```python
from build123d import *

# Parameters (mm, degrees)
CROQUIS1_R     = 11
CROQUIS1_R_2   = 4
EXTRUIR1_DEPTH = 0.7
CROQUIS2_R     = 11
CROQUIS2_R_2   = 10.3
CROQUIS2_R_3   = 8.9
CROQUIS2_R_4   = 8.2
CROQUIS2_R_5   = 6.8
CROQUIS2_R_6   = 6.1
CROQUIS2_R_7   = 4.7
CROQUIS2_R_8   = 4
EXTRUIR2_DEPTH = 1.6
CROQUIS3_R     = 4.7
CROQUIS3_R_2   = 4
EXTRUIR3_DEPTH = 0.7


with BuildPart() as part:
    # Croquis1 → Extruir1 (new body)
    with BuildSketch(Plane(origin=(0, 0, 0), x_dir=(1, 0, 0), z_dir=(0, 1, 0))):
        with Locations(Location((0, 0, 0), (0, 0, 270))):
            Circle(CROQUIS1_R)
        with Locations(Location((0, 0, 0), (0, 0, 270))):
            Circle(CROQUIS1_R_2, mode=Mode.SUBTRACT)
    extrude(amount=EXTRUIR1_DEPTH)

    # Croquis2 → Extruir2 (add)
    # profile 1 of 4: a face of its own
    with BuildSketch(Plane(origin=(0, 0.7, 0), x_dir=(1, 0, 0), z_dir=(0, 1, 0))):
        with Locations(Location((0, 0, 0), (0, 0, 270))):
            Circle(CROQUIS2_R)
        with Locations(Location((0, 0, 0), (0, 0, 270))):
            Circle(CROQUIS2_R_2, mode=Mode.SUBTRACT)
    # profile 2 of 4: a face of its own
    with BuildSketch(Plane(origin=(0, 0.7, 0), x_dir=(1, 0, 0), z_dir=(0, 1, 0))):
        with Locations(Location((0, 0, 0), (0, 0, 270))):
            Circle(CROQUIS2_R_3)
        with Locations(Location((0, 0, 0), (0, 0, 270))):
            Circle(CROQUIS2_R_4, mode=Mode.SUBTRACT)
    # profile 3 of 4: a face of its own
    with BuildSketch(Plane(origin=(0, 0.7, 0), x_dir=(1, 0, 0), z_dir=(0, 1, 0))):
        with Locations(Location((0, 0, 0), (0, 0, 270))):
            Circle(CROQUIS2_R_5)
        with Locations(Location((0, 0, 0), (0, 0, 270))):
            Circle(CROQUIS2_R_6, mode=Mode.SUBTRACT)
    # profile 4 of 4: a face of its own
    with BuildSketch(Plane(origin=(0, 0.7, 0), x_dir=(1, 0, 0), z_dir=(0, 1, 0))):
        with Locations(Location((0, 0, 0), (0, 0, 270))):
            Circle(CROQUIS2_R_7)
        with Locations(Location((0, 0, 0), (0, 0, 270))):
            Circle(CROQUIS2_R_8, mode=Mode.SUBTRACT)
    extrude(amount=EXTRUIR2_DEPTH)

    # Croquis3 → Extruir3 (add)
    with BuildSketch(Plane(origin=(0, 2.3, 0), x_dir=(1, 0, 0), z_dir=(0, 1, 0))):
        with Locations(Location((0, 0, 0), (0, 0, 270))):
            Circle(CROQUIS3_R)
        with Locations(Location((0, 0, 0), (0, 0, 270))):
            Circle(CROQUIS3_R_2, mode=Mode.SUBTRACT)
    extrude(amount=EXTRUIR3_DEPTH)


solid = part.part
```
Check sheet for the modelled part. Datum: model origin and axes. Units: mm. A direction names the side the tool comes from. Coordinates: 2 decimals unless noted, no trailing zeros. Loops run counter-clockwise (first coordinate to the right, second up) from the corner with the lowest first, then second, coordinate; pieces in that order, holes last.
1) Access from +Z, -Z, +X, -X, +Y, -Y to the whole of each face (thin tool, end or side, straight path). Record for faces 4 (the face through (-5, 0, 0)), 5 (the face through (7, 0.7, 1)).
2) Release check for a two-part mould opening along X. For faces 1 (the face through (4, 3, 2)), 2 (the face through (-10.74, 1.13, -2.38)), 3 (the face through (1.412, 1.834, 4.483)) record: released by +X, released by -X, zero draft, split by the parting line, or undercut.
3) Material ranges on probe 1 along X at (y, z) = (1.05, -6.25); probe 2 along X at (y, z) = (1.15, 7.25); probe 3 along X at (y, z) = (1.2, -5.25), recorded low to high.
4) Gauge pin test, flat ends, axial feed: pin 1 (1 mm diameter, centred on x = 2, y = 0.5, fed in from -Z); pin 2 (7 mm diameter, centred on x = 0, z = 0, fed in from -Y); pin 3 (1 mm diameter, centred on x = -5, y = 2.5, fed in from -Z). Record the tip position at first contact, or that the pin passes through.
5) Sectioned sample at A-A (y = 1.05). Record the boundary of the cut face in (x, z).
6) Sectioned sample at D-D (x = 8.5). Record the boundary of the cut face in (y, z).
Check sheet entries:
1. face 4: +Z, -Z, +X, -X, -Y
1. face 5: +Y
2. face 1: zero draft
2. face 2: split by the parting line
2. face 3: undercut
3. probe 1: x = -9.05 to -8.19, -6.34 to -5.31, -2.68 to 2.68, 5.31 to 6.34, 8.19 to 9.05
3. probe 2: x = -8.27 to -7.32, -5.16 to -3.83, 3.83 to 5.16, 7.32 to 8.27
3. probe 3: x = -9.67 to -8.86, -7.19 to -6.3, -4.32 to -3.11, 3.11 to 4.32, 6.3 to 7.19, 8.86 to 9.67
4. pin 1: stops at z = -10.9
4. pin 2: passes through
4. pin 3: stops at z = -10.02
5. outline: circle Ø22 at (0, 0); circle Ø17.8 at (0, 0); circle Ø13.6 at (0, 0); circle Ø9.4 at (0, 0); hole circle Ø20.6 at (0, 0); hole circle Ø16.4 at (0, 0); hole circle Ø12.2 at (0, 0); hole circle Ø8 at (0, 0)
6. outline: (0, -6.98) - (2.3, -6.98) - (2.3, -5.82) - (0.7, -5.82) - (0.7, -2.64) - (2.3, -2.64) - (2.3, 2.64) - (0.7, 2.64) - (0.7, 5.82) - (2.3, 5.82) - (2.3, 6.98) - (0, 6.98) - close
